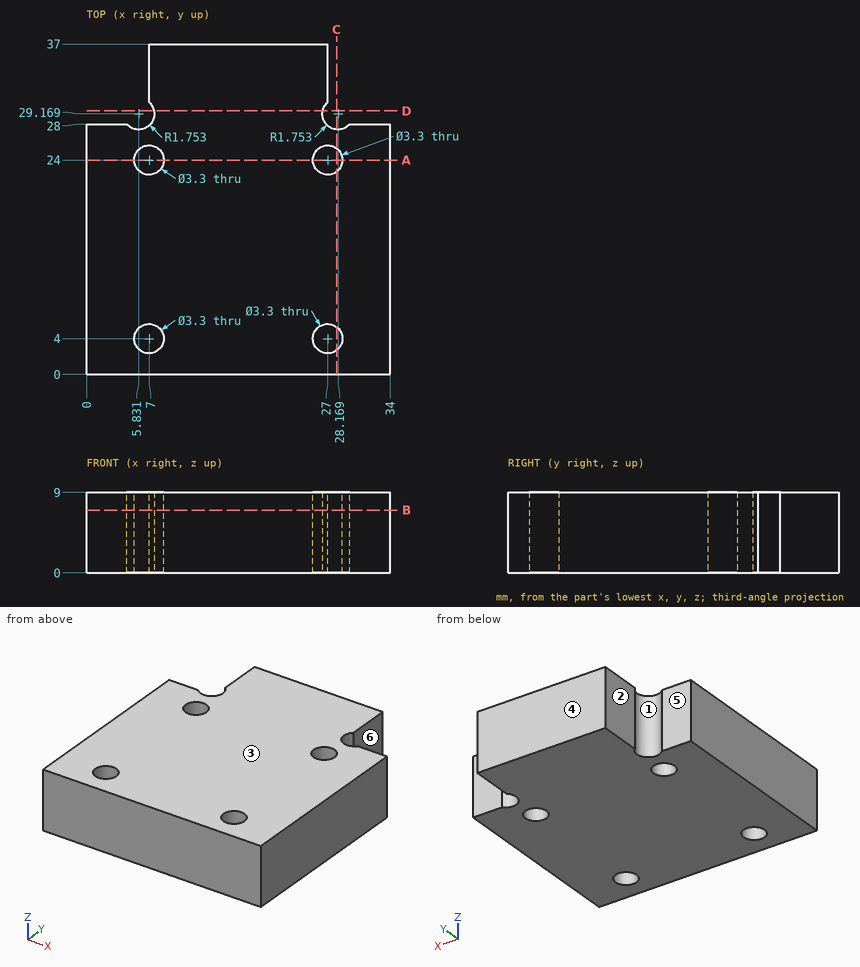
Here's the drawing with two shaded views (mm, measured from the low corner). I have some questions. A direction names the side the tool comes from. Give positions to 0.01 mm unless a question says otherwise; leave off trailing zeros. Order: outer loops, then holes, each group sorted by start corner. A loop starts at its lowest first (then second) coordinate and runs counter-clockwise, first axis right, second up. Notation, with made-up numbers: M 22.25,-34 L 69.25,-34 A15 cw 69.25,-29 Z; hole C -36,6 d7. An arc over 180 degrees is marked long. Answer as a JSON object with one key per item and string values. Group by question number.
1) On a 3-axis mill with a long thin cutter (end or side, diameter ignored), from which of +Z, -Z, +X, -X, +Y, -Y can I reach the whole of each face in a straight line? I mean the marked faces 4, 5 and 6. Say none if no direction works.
2) Suppose I cut it at B-B, the plane z = 7. Count the separate pieces of the cut face and the enclosed holes in it, plus the area to 3 significant figures.
3) Suppose I cut it at C-C, the plane x = 28. Write out the boundary of the cut face in (y, z).
4) Suppose I cut it at A-A, the plane y = 24. Write out the boundary of the cut face in (x, z).
5) We'd pull the mould along X, two halves only. Please class the marked faces 1, 2 and 3: pulls with the +X half, pulls with the -X half, needs draft (parallel to the pull), parting line crosses it, or undercut.
6) I'm going to push flat-ended pins straight in: pin 1 Ø2 at (x, y) = (7, 24) entering from -Z; pin 2 Ø2 at (y, z) = (32.5, 4) entering from -X; pin 3 Ø2 at (x, y) = (10, 5.5) entering from -Z; pin 4 Ø2 at (y, z) = (34.5, 5.5) entering from +X. Where does each tip first touch, or does it pass through?
7) Please list where these lines run through material, in increasing order: L1, parallel to X at y = 23.5, z = 6.25; L2, parallel to X at y = 5, z = 7.75; L3, parallel to Y at x = 8, z = 1.25. Write a range as [from, to].
8) Suppose I cut it at D-D, the plane y = 29.5. Write out the boundary of the cut face in (x, z), plus the area to 3 significant figures.
Results found:
{
 "1": {"face 4": "+Z, -Z, +X, -X, +Y", "face 5": "+Z, -Z, -X, +Y", "face 6": "+Z, -Z, +X, +Y"},
 "2": {"separate pieces": "1", "enclosed holes": "4", "area": "1,090 mm²"},
 "3": {"outline": "M 0,0 L 2.69,0 L 2.69,9 L 0,9 Z; M 5.31,0 L 22.69,0 L 22.69,9 L 5.31,9 Z; M 25.31,0 L 27.42,0 L 27.42,9 L 25.31,9 Z"},
 "4": {"outline": "M 0,0 L 5.35,0 L 5.35,9 L 0,9 Z; M 8.65,0 L 25.35,0 L 25.35,9 L 8.65,9 Z; M 28.65,0 L 34,0 L 34,9 L 28.65,9 Z"},
 "5": {"face 1": "undercut", "face 2": "pulls with the -X half", "face 3": "needs draft"},
 "6": {"pin 1": "through", "pin 2": "x = 7", "pin 3": "z = 0", "pin 4": "x = 27"},
 "7": {"L1": "[0, 5.43], [8.57, 25.43], [28.57, 34]", "L2": "[0, 5.69], [8.31, 25.69], [28.31, 34]", "L3": "[0, 2.69], [5.31, 22.69], [25.31, 37]"},
 "8": {"outline": "M 7.55,0 L 26.45,0 L 26.45,9 L 7.55,9 Z", "area": "170 mm²"}
}
